```python
from build123d import *

# Parameters (mm, degrees)
BOSS_EXTRUDE1_DEPTH = 6


with BuildPart() as part:
    # Sketch1 → Boss-Extrude1 (new body)
    with BuildSketch(Plane.XY):
        with BuildLine():
            Line((-6, 0), (-6, -494.15))
            ThreePointArc((-6, -494.15), (-4.242640687, -498.392640687), (0, -500.15))
            Line((0, -500.15), (402, -500.15))
            ThreePointArc((402, -500.15), (406.242640687, -498.392640687), (408, -494.15))
            Line((408, -494.15), (408, -119.649819196))
            ThreePointArc((408, -119.649819196), (406.242640687, -115.407178509), (402, -113.649819196))
            Line((402, -113.649819196), (77.763956729, -113.649819196))
            ThreePointArc((77.763956729, -113.649819196), (73.509598553, -111.877262252), (71.772388716, -107.60834862))
            ThreePointArc((71.772388716, -107.60834862), (73.251375418, -104.099653504), (76.772216732, -102.649819196))
            Line((76.772216732, -102.649819196), (84.272216732, -102.649819196))
            Line((84.272216732, -102.649819196), (84.272216732, -104.149819196))
            Line((84.272216732, -104.149819196), (76.772216732, -104.149819196))
            ThreePointArc((76.772216732, -104.149819196), (74.343547137, -105.129588254), (73.274612012, -107.520354054))
            ThreePointArc((73.274612012, -107.520354054), (74.521274443, -110.783312955), (77.735886194, -112.149819196))
            Line((77.735886194, -112.149819196), (402, -112.149819196))
            ThreePointArc((402, -112.149819196), (407.303300859, -114.346518337), (409.5, -119.649819196))
            Line((409.5, -119.649819196), (409.5, -494.15))
            ThreePointArc((409.5, -494.15), (407.303300859, -499.453300859), (402, -501.65))
            Line((402, -501.65), (0, -501.65))
            ThreePointArc((0, -501.65), (-5.303300859, -499.453300859), (-7.5, -494.15))
            Line((-7.5, -494.15), (-7.5, 0))
            ThreePointArc((-7.5, 0), (0, 7.5), (7.5, 0))
            Line((7.5, 0), (7.5, -106.149819196))
            ThreePointArc((7.5, -106.149819196), (9.257359313, -110.392459883), (13.5, -112.149819196))
            Line((13.5, -112.149819196), (57.772216732, -112.149819196))
            ThreePointArc((57.772216732, -112.149819196), (61.772216732, -108.149819196), (57.772216732, -104.149819196))
            Line((57.772216732, -104.149819196), (50.272216732, -104.149819196))
            Line((50.272216732, -104.149819196), (50.272216732, -102.649819196))
            Line((50.272216732, -102.649819196), (57.772216732, -102.649819196))
            ThreePointArc((57.772216732, -102.649819196), (63.272216732, -108.149819196), (57.772216732, -113.649819196))
            Line((57.772216732, -113.649819196), (13.5, -113.649819196))
            ThreePointArc((13.5, -113.649819196), (8.196699141, -111.453120055), (6, -106.149819196))
            Line((6, -106.149819196), (6, 0))
            ThreePointArc((6, 0), (0, 6), (-6, 0))
        make_face()
    extrude(amount=BOSS_EXTRUDE1_DEPTH)


solid = part.part
```
Geometry check sheet. Reference: the model listing, model coordinates, mm. Coordinates: 2 decimals unless noted, no trailing zeros. Loops run counter-clockwise (first coordinate to the right, second up) from the corner with the lowest first, then second, coordinate; pieces in that order, holes last. Notation, with made-up numbers: (72, -2) - (82, -2) arc R12 ccw to (82, 18) - close; hole circle Ø11 at (38, 78.5). An arc over 180 degrees is marked (long way). One line per item, written item: value. Start each with the question number.
(1) Material ranges on line 1 (X direction, y = -194, z = 0.8); line 2 (X direction, y = -14, z = 1.35); line 3 (Y direction, x = 30, z = 4.5), recorded low to high. Write a range as [from, to].
(2) Cross-section at B-B on x = 130.5. Enter the section's corners in (y, z).
(3) Depth check by flat-ended pin: P1, Ø8, axis at x = 86.5, y = -96, coming from the -Z side; P2, Ø1.2, axis at y = -103.5, z = 4.5, coming from the +X side; P3, Ø3, axis at y = -57.5, z = 4, coming from the +X side; P4, Ø3, axis at x = 53.5, z = 2, coming from the +Y side. Enter the tip coordinate at first touch or a pass-through.
(4) Cross-section at A-A on y = -151. Enter the section's corners in (x, z).
Results below:
1. line 1: x = [-7.5, -6], [408, 409.5]
1. line 2: x = [-7.5, -6], [6, 7.5]
1. line 3: y = [-501.65, -500.15], [-113.65, -112.15]
2. outline: (-501.65, 0) - (-500.15, 0) - (-500.15, 6) - (-501.65, 6) - close; (-113.65, 0) - (-112.15, 0) - (-112.15, 6) - (-113.65, 6) - close
3. P1: passes through
3. P2: stops at x = 84.27
3. P3: stops at x = 7.5
3. P4: stops at y = -102.65
4. outline: (-7.5, 0) - (-6, 0) - (-6, 6) - (-7.5, 6) - close; (408, 0) - (409.5, 0) - (409.5, 6) - (408, 6) - close
